Input: part model. Units: mm. Frame: model coordinates. A direction names the side the tool comes from. Give positions to 0.01 mm unless a question says otherwise; leave off trailing zeros. Loops run counter-clockwise (first coordinate to the right, second up) from the corner with the lowest first, then second, coordinate; pieces in that order, holes last. Notation, with made-up numbers: M 24.25,17 L 31.25,17 A20 ccw 31.25,51 Z; hole C -33.5,71.25 d4. An arc over 180 degrees is marked long. Answer as a JSON object with one key per item and string values. Group by question number.
```python
from build123d import *

# Parameters (mm, degrees)
F0_R          = 7.6
F1_DEPTH      = 12
F2_R          = 7.6
F3_DEPTH      = 2.6
F4_R          = 1.4
F5_DEPTH      = 12.001
F6_R          = 10
F7_DEPTH      = 90
F8_R          = 1.4
F9_DEPTH      = 17.601
F9_DEPTH_BACK = 167.601


with BuildPart() as f1:
    # F0 (on Top) → F1 (new body)
    with BuildSketch(Plane.XY):
        with BuildLine():
            ThreePointArc((16.6522889532, -5.697479497), (17.3614556644, -2.8878810938), (17.6, 0))
            ThreePointArc((17.6, 0), (-2.8878810938, 17.3614556644), (-16.6522889532, -5.697479497))
            ThreePointArc((-16.6522889532, -5.697479497), (0, -17.6), (16.6522889532, -5.697479497))
        make_face()
        Circle(F0_R, mode=Mode.SUBTRACT)
        with BuildLine():
            ThreePointArc((16.6522889532, -5.697479497), (0, -17.6), (-16.6522889532, -5.697479497))
            ThreePointArc((-16.6522889532, -5.697479497), (-5.1246012651, -75), (-16.6522889532, -144.302520503))
            ThreePointArc((-16.6522889532, -144.302520503), (0, -132.4), (16.6522889532, -144.302520503))
            ThreePointArc((16.6522889532, -144.302520503), (5.1246012651, -75), (16.6522889532, -5.697479497))
        make_face()
        with BuildLine():
            ThreePointArc((16.6522889532, -144.302520503), (0, -132.4), (-16.6522889532, -144.302520503))
            ThreePointArc((-16.6522889532, -144.302520503), (-2.8878810938, -167.3614556644), (17.6, -150))
            ThreePointArc((17.6, -150), (17.3614556644, -147.1121189062), (16.6522889532, -144.302520503))
        make_face()
        Circle(F0_R)
    extrude(amount=F1_DEPTH)

    # F2 (on Top) → F3 (cut)
    with BuildSketch(Plane.XY):
        Circle(F2_R)
        with Locations((0, -150)):
            Circle(F2_R)
    extrude(amount=F3_DEPTH, mode=Mode.SUBTRACT)

    # F4 (on Top) → F5 (cut, through all)
    with BuildSketch(Plane.XY):
        with Locations((0, -150)):
            Circle(F4_R)
        Circle(F4_R)
    extrude(amount=F5_DEPTH, mode=Mode.SUBTRACT)

    # F6 (on face) → F7 (join)
    with BuildSketch(Plane.XY.offset(12)):
        Circle(F6_R)
    extrude(amount=F7_DEPTH)

    # F8 (on Front) → F9 (cut, two sides)
    with BuildSketch(Plane.XZ) as f9_sk:
        with Locations((0, 97)):
            Circle(F8_R)
    extrude(amount=-F9_DEPTH, mode=Mode.SUBTRACT)
    extrude(f9_sk.sketch, amount=F9_DEPTH_BACK, mode=Mode.SUBTRACT)


solid = f1.part
```
1. First-contact query: P1, Ø2, axis at x = 0, y = -150, coming from the -Z side; P2, Ø5, axis at x = 2.5, y = -58, coming from the +Z side; P3, Ø12, axis at x = -1, y = -149.5, coming from the -Z side; P4, Ø0.8, axis at x = 0, y = 0, coming from the -Z side. Flat tips, straight axial feed; report the tip coordinate or a pass-through.
2. Section B-B (z = 74.5). Output: boundary loops of the cut face in (x, y), then the cut area to 3 significant figures.
3. Material intervals for L1, parallel to Y at x = 0, z = 8; L2, parallel to Z at x = 0, y = 7.25; L3, parallel to Z at x = 6, y = -115.5, sorted ascending.
4. Reachability of faces 4 (the flat face through (0, -74, 0)), 5 (the cylindrical face through (-1.65, -157.42, 1.28)) from +Z, -Z, +X, -X, +Y, -Y: full face, straight path, thin tool, end or side. Return the list, or none.
5. Section D-D (y = -17). Output: boundary loops of the cut face in (x, z), then the cut area to 3 significant figures.
6. Section C-C (y = -97). Output: boundary loops of the cut face in (x, z), then the cut area to 3 significant figures.
7. Section A-A (x = -13.5). Output: boundary loops of the cut face in (y, z), then the cut area to 3 significant figures.
8. Mould query, pull axis X, two halves, no side actions, for faces 1 (the cylindrical face through (5.127, -75.988, 5.916)), 2 (the flat face through (0, -152, 2.6)), 3 (the cylindrical face through (-2.17, -9.76, 56.37)). Classes: pulls with the +X half, pulls with the -X half, needs draft (parallel to the pull), parting line crosses it, or undercut.
Geometry results:
{
 "1": {"P1": "through", "P2": "z = 12", "P3": "z = 2.6", "P4": "z = 12"},
 "2": {"outline": "C 0,0 d20", "area": "314 mm2"},
 "3": {"L1": "-167.6 to -151.4, -148.6 to -1.4, 1.4 to 17.6", "L2": "2.6 to 95.6, 98.4 to 102", "L3": "0 to 12"},
 "4": {"face 4": "-Z, +X, -X, +Y, -Y", "face 5": "-Z"},
 "5": {"outline": "M -13.13,0 L 13.13,0 L 13.13,12 L -13.13,12 Z", "area": "315 mm2"},
 "6": {"outline": "M -6.26,0 L 6.26,0 L 6.26,12 L -6.26,12 Z", "area": "150 mm2"},
 "7": {"outline": "M -161.29,0 L -134.29,0 L -134.29,12 L -161.29,12 Z; M -15.71,0 L 11.29,0 L 11.29,12 L -15.71,12 Z", "area": "648 mm2"},
 "8": {"face 1": "pulls with the +X half", "face 2": "undercut", "face 3": "parting line crosses it"}
}
